Autodesk Inventor part; units mm, degrees
ref_plane "YZ Plane" through (0, 0, 0) normal (1, 0, 0) x (0, 1, 0)
ref_plane "XZ Plane" through (0, 0, 0) normal (0, 1, 0) x (-1, 0, 0)
ref_plane "XY Plane" through (0, 0, 0) normal (0, 0, 1) x (1, 0, 0)
sketch "Sketch1" plane through (0, 0, 0) normal (0, 1, 0) x (-1, 0, 0)
  circle A0 centre (0, 0) radius 1.5
  circle A1 centre (0, 0) radius 5
  line L0 (-5, 0) -> (-5, 5)
  line L1 (-5, 5) -> (0, 5)
  line L2 (-5, 0) -> (-5, -20)
  line L3 (-5, -20) -> (-1.5, -20)
  line L4 (-5, -20) -> (0, -20)
  line L5 (0, -20) -> (0, -5)
  dimension "d0" = 3
  dimension "d1" = 10
  dimension "d2" = 20
extrude "Extrusion1" add sketch "Sketch1" along normal blind 7
sketch "Sketch2" plane through (5, 0, 5) normal (1, 0, 0) x (0, 0, -1)
  line L0 (10, 7) -> (0, 7)
  line L1 (0, 7) -> (0, 3.5)
  line L2 (0, 0) -> (25, 0)
  line L3 (0, 3.5) -> (5, 3.5)
  circle A0 centre (5, 3.5) radius 3
  point P0 (5, 0)
  dimension "d5" = 3.5
  dimension "d6" = 6
extrude "Extrusion2" add sketch "Sketch2" along normal blind 15
sketch "Sketch3" plane through (5, 0, 5) normal (1, 0, 0) x (0, 0, -1)
  point P0 (5, 0)
sketch "Sketch7" plane through (0, 7, 0) normal (0, 1, 0) x (1, 0, 0)
  line L0 (0, 19.9362) -> (0, 16.9362)
  line L1 (0, 20) -> (0, 5)
  line L2 (0, 16.9362) -> (-1.5, 16.9362)
  circle A0 centre (-1.5, 16.9362) radius 1.5
  circle A1 centre (-1.5, 16.9362) radius 3.4113
  point P0 (0, 0)
  point P1 (0, 13.8723)
  dimension "d25" = 3
  dimension "d26" = 1.5
extrude "Extrusion6" add sketch "Sketch7" against normal blind 7 contours L0 L1 A1 picked at (-0.578, 19.5142)
sketch "Sketch8" plane through (0, 0, -5) normal (-1, 0, 0) x (0, 0, 1)
  line L0 (-8.8723, 7) -> (0, 7)
  line L1 (-7.6834, 7) -> (-4.1834, 7)
  line L2 (-7.6834, 7) -> (-7.6834, 3.5)
  line L3 (-7.6834, 7) -> (-4.1834, 7) construction
  line L4 (-7.6834, 3.5) -> (-7.6834, 1.8)
  line L5 (-7.6834, 1.8) -> (-17.6834, 1.8)
  line L6 (-17.6834, 1.8) -> (-17.6834, 5.2)
  line L7 (-17.6834, 5.2) -> (-7.6834, 5.2)
  line L8 (-7.6834, 5.2) -> (-7.6834, 1.8)
  point P0 (5, 0)
  point P1 (-7.6834, 5.2)
  dimension "d29" = 3.5
  dimension "d30" = 3.5
  dimension "d31" = 90
  dimension "d32" = 1.7
  dimension "d33" = 10
  dimension "d34" = 3.4
extrude "Extrusion7" cut sketch "Sketch8" along normal blind 7
properties part number "stuur_ARMPJE"
Geometry check sheet. Reference: the model listing, model coordinates, mm. A direction names the side the tool comes from. Round coordinates to 2 decimals unless told otherwise and drop trailing zeros. Loops run counter-clockwise (first coordinate to the right, second up) from the corner with the lowest first, then second, coordinate; pieces in that order, holes last. Notation, with made-up numbers: M 42,34 L 78,34 A34 cw 78,65 Z; hole C 28.5,-24.5 d6. An arc over 180 degrees is marked long. Return JSON: item names as keys, results as strings. Group by question number.
(1) Section check B-B, the plane z = 0. Enter the section's corners in (x, y), and give its area (3 significant figures).
(2) Section check D-D, the plane x = 16.75. Enter the section's corners in (y, z).
(3) Section check A-A, the plane y = 3.5. Enter the section's corners in (x, z), and give its area (3 significant figures).
(4) Mould release check, pull along X, two halves, no side actions. Record for faces 4 (the face through (20, 4, 0)), 5 (the face through (12.4, 3.4, 3)), 6 (the face through (-1.825, 6.113, -15.472)): pulls with the +X half, pulls with the -X half, needs draft (parallel to the pull), parting line crosses it, or undercut.
(5) Section check C-C, the plane y = 5.75. Enter the section's corners in (x, z).
(6) Set-up check for faces 1 (the face through (1, 7, -8)), 2 (the face through (3, 3, -20)), 3 (the face through (-3, 5.2, -16)): record each of +Z, -Z, +X, -X, +Y, -Y from which the full face is reachable in a straight line by a thin tool's end or side.
(7) Go/stop test with flat-tipped pins: pin 1 (5.5 mm diameter, centred on x = -3.5, z = -16.5, fed in from -Y); pin 2 (2 mm diameter, centred on x = 11.5, y = 1.5, fed in from -Z); pin 3 (1 mm diameter, centred on y = 4, z = -16, fed in from +X); pin 4 (1.5 mm diameter, centred on x = 2, y = 3, fed in from -Z). Record where each tip stops, or that it passes through.
(8) Scan lines: line 1 along Z through (x, y) = (-0.5, 6.75); line 2 along X through (y, z) = (2.75, -18.5); line 3 along Y through (x, z) = (14.75, 0). Record each from-to range of solid material in increasing order. Write a range as [from, to].
Data:
{
 "1": {"outline": "M -5,0 L -1.5,0 L -1.5,7 L -5,7 Z; M 1.5,0 L 5,0 L 5,0.5 L 20,0.5 L 20,6.5 L 5,6.5 L 5,7 L 1.5,7 Z", "area": "139 mm²"},
 "2": {"outline": "C 3.5,0 d6"},
 "3": {"outline": "M 0,-20 L 5,-20 L 5,-3 L 20,-3 L 20,3 L 5,3 L 5,5 L 0,5 A5 ccw 0,-5 Z; hole C 0,0 d3", "area": "247 mm²"},
 "4": {"face 4": "pulls with the +X half", "face 5": "needs draft", "face 6": "undercut"},
 "5": {"outline": "M 0,-20 L 5,-20 L 5,-1.98 L 20,-1.98 L 20,1.98 L 5,1.98 L 5,5 L 0,5 A5 ccw 0,-5 L 0,-13.87 A3.41 ccw long Z; hole C -1.5,-16.94 d3; hole C 0,0 d3"},
 "6": {"face 1": "+Z, -Z, +X, -X, +Y", "face 2": "-Z, +X, +Y, -Y", "face 3": "-Z, -X"},
 "7": {"pin 1": "y = 0", "pin 2": "z = -2.83", "pin 3": "x = 5", "pin 4": "z = -20"},
 "8": {"line 1": "[-20.2, -18.05], [-15.82, -13.67], [-4.97, -1.41], [1.41, 4.97]", "line 2": "[0, 5]", "line 3": "[0.5, 6.5]"}
}
